from build123d import *

# Parameters (mm, degrees)
PAD_DEPTH       = 50
POCKET_DEPTH    = 15
SKETCH003_R     = 2.2
POCKET002_DEPTH = 20.001
SKETCH004_W     = 2.6
SKETCH004_H     = 8.1
POCKET003_DEPTH = 10.5
SKETCH005_R     = 4
POCKET004_DEPTH = 6
SKETCH002_R     = 2.75
POCKET005_DEPTH = 45


with BuildPart() as part:
    # Sketch → Pad (new body)
    with BuildSketch(Plane.XZ):
        Polygon((0, 0), (65, 0), (65, 12), (10, 12), (12.143594, 20), (0, 20), align=None)
    extrude(amount=PAD_DEPTH)

    # Sketch001 (on Face2 of Pad) → Pocket (cut)
    with BuildSketch(Plane(origin=(65, 0, 0), x_dir=(0, 0, 1), z_dir=(1, 0, 0))):
        Polygon((0, 32.5), (12, 40), (12, 10), (0, 17.5), (0, 25), align=None)
    extrude(amount=-POCKET_DEPTH, mode=Mode.SUBTRACT)

    # Sketch003 → Pocket002 (cut, through all)
    with BuildSketch(Plane(origin=(0, 0, 0), x_dir=(1, 0, 0), z_dir=(0, 0, -1))):
        with Locations((32.5, 35)):
            Circle(SKETCH003_R)
        with Locations((32.5, 15)):
            Circle(SKETCH003_R)
    extrude(amount=-POCKET002_DEPTH, mode=Mode.SUBTRACT)

    # Sketch004 (on Face12 of Pocket002) → Pocket003 (cut)
    with BuildSketch(Plane(origin=(0, 0, 12), x_dir=(-1, 0, 0), z_dir=(0, 0, 1))):
        with Locations((-35, 25)):
            Rectangle(SKETCH004_W, SKETCH004_H)
    extrude(amount=-POCKET003_DEPTH, mode=Mode.SUBTRACT)

    # Sketch005 (on Face12 of Pocket003) → Pocket004 (cut)
    with BuildSketch(Plane(origin=(0, 0, 12), x_dir=(-1, 0, 0), z_dir=(0, 0, 1))):
        with Locations((-32.5, 35)):
            Circle(SKETCH005_R)
        with Locations((-32.5, 15)):
            Circle(SKETCH005_R)
    extrude(amount=-POCKET004_DEPTH, mode=Mode.SUBTRACT)

    # Sketch002 (on Face5 of Pocket) → Pocket005 (cut)
    with BuildSketch(Plane(origin=(50, 0, 0), x_dir=(0, 0, 1), z_dir=(1, 0, 0))):
        with Locations((6, 25)):
            Circle(SKETCH002_R)
    extrude(amount=-POCKET005_DEPTH, mode=Mode.SUBTRACT)


solid = part.part
Design review of the part built by this model. Coordinates are the model's own, in mm. A direction names the side the tool comes from. Give positions to 0.01 mm unless a question says otherwise; leave off trailing zeros. Loops run counter-clockwise (first coordinate to the right, second up) from the corner with the lowest first, then second, coordinate; pieces in that order, holes last. Notation, with made-up numbers: (32, -39.5) - (68, -39.5) arc R12 ccw to (68, -26.5) - close; hole circle Ø1 at (14.25, 51.25). An arc over 180 degrees is marked (long way). Write item = value, one per line.
1) Take a section at B-B on y = -35. State the section outline as (x, z) points, and give its area (3 significant figures).
Result sheet:
outline = (0, 0) - (30.3, 0) - (30.3, 6) - (28.5, 6) - (28.5, 12) - (10, 12) - (12.14, 20) - (0, 20) - close; (34.7, 0) - (65, 0) - (65, 4) - (50, 4) - (50, 12) - (36.5, 12) - (36.5, 6) - (34.7, 6) - close
area = 674 mm2
2) Tool access review of faces 5 (the face through (5, -25, 6)), 6 (the face through (57.6, -36.2, 5.92)), 7 (the face through (33.7, -25, 9)): name each direction out of +Z, -Z, +X, -X, +Y, -Y from which nothing blocks a thin tool from reaching the whole face with its end or side.
Result sheet:
face_5 = +X
face_6 = +Z, +X
face_7 = +Z
3) Clearance check with flat-ended pins moving along their axes: pin 1 Ø4.5 at (y, z) = (-25, 6) entering from +X; pin 2 Ø6.5 at (x, y) = (30.5, -14) entering from +Z; pin 3 Ø6 at (y, z) = (-28.5, 7) entering from +X; pin 4 Ø5 at (x, z) = (29, 15.5) entering from -Y. State where each tip first meets the part, or that it passes through.
Result sheet:
pin_1 = 5
pin_2 = 12
pin_3 = 50
pin_4 = through
4) Take a section at A-A on x = 32.5. State the section outline as (y, z) points, and give its area (3 significant figures).
Result sheet:
outline = (-50, 0) - (-37.2, 0) - (-37.2, 6) - (-39, 6) - (-39, 12) - (-50, 12) - close; (-32.8, 0) - (-17.2, 0) - (-17.2, 6) - (-19, 6) - (-19, 12) - (-31, 12) - (-31, 6) - (-32.8, 6) - close; (-12.8, 0) - (0, 0) - (0, 12) - (-11, 12) - (-11, 6) - (-12.8, 6) - close; hole circle Ø5.5 at (-25, 6)
area = 427 mm2
5) Take a section at C-C on x = 59.5. State the section outline as (y, z) points, and give its area (3 significant figures).
Result sheet:
outline = (-50, 0) - (-32.5, 0) - (-40, 12) - (-50, 12) - close; (-17.5, 0) - (0, 0) - (0, 12) - (-10, 12) - close
area = 330 mm2
6) Draft analysis for pull direction Y (two halves, no side actions). For faces 1 (the face through (11.057, -24.65, 15.944)), 2 (the face through (35.45, -17.7, 9.04)), 3 (the face through (32, 0, 8)), 4 (the face through (31, -13, 6)), state which applies: +Y half, -Y half, draft (parallel to the pull), parting line (faces both ways), or undercut.
Result sheet:
face_1 = draft
face_2 = undercut
face_3 = +Y half
face_4 = undercut
7) To check wall thickness, follow line 1 (X direction, y = -35, z = 3.9); line 2 (Z direction, x = 16, y = -25); line 3 (Y direction, x = 35, z = 9). State the ranges of each line that lie inside material, in increasing order.
Result sheet:
line_1 = 0 to 30.3, 34.7 to 65
line_2 = 0 to 3.25, 8.75 to 12
line_3 = -50 to -38.12, -31.88 to -29.05, -20.95 to -18.12, -11.88 to 0
8) Take a section at D-D on z = 8. State the section outline as (x, y) points, and give its area (3 significant figures).
Result sheet:
outline = (0, -50) - (65, -50) - (65, -37.5) - (50, -37.5) - (50, -26.89) - (36.3, -26.89) - (36.3, -29.05) - (33.7, -29.05) - (33.7, -26.89) - (5, -26.89) - (5, -23.11) - (33.7, -23.11) - (33.7, -20.95) - (36.3, -20.95) - (36.3, -23.11) - (50, -23.11) - (50, -12.5) - (65, -12.5) - (65, 0) - (0, 0) - close; hole circle Ø8 at (32.5, -35); hole circle Ø8 at (32.5, -15)
area = 2,590 mm2
